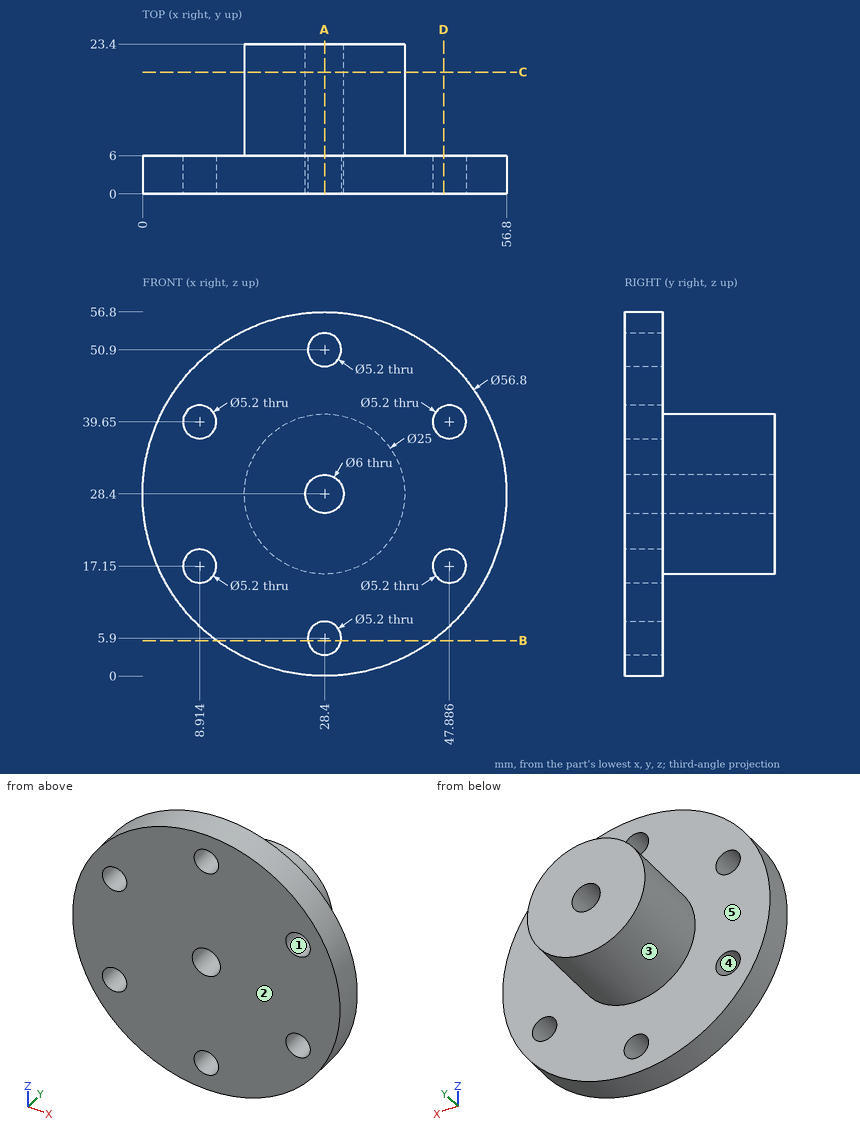
Part print with two shaded views. Sizes in mm from the minimum x, y, z corner. A direction names the side the tool comes from. Round coordinates to 2 decimals unless told otherwise and drop trailing zeros. Loops run counter-clockwise (first coordinate to the right, second up) from the corner with the lowest first, then second, coordinate; pieces in that order, holes last. Notation, with made-up numbers: M 57,23 L 69,23 A14 cw 69,44 Z; hole C -27.5,19 d5. An arc over 180 degrees is marked long. Put each result on its own line as item: value. Start each with the question number.
Item 1: Drop flat-ended pins along their axis: P1, Ø4, axis at y = 3.5, z = 23.5, coming from the -X side; P2, Ø1.5, axis at y = 6.5, z = 38.5, coming from the -X side; P3, Ø6, axis at x = 22, y = 14.5, coming from the -Z side. Give the stop position or say it passes through.
Item 2: Cut at B-B (z = 5.5). List the corners of the cut face in (x, y).
Item 3: Cut at D-D (x = 47). List the corners of the cut face in (y, z) (1 decimal), then the cut area to 3 significant figures.
Item 4: Cut at C-C (y = 19). List the corners of the cut face in (x, z).
Item 5: Mould opens along X. For the marked faces 1, 2 and 3 say: released by +X, released by -X, zero draft, split by the parting line, or undercut.
Item 6: Cut at A-A (x = 28.4). List the corners of the cut face in (y, z), then the cut area to 3 significant figures.
Item 7: Drill centre lines: line 1 along X through (y, z) = (1.4, 17.15) (1 decimal); line 2 along Z through (x, y) = (8.5, 4.5) (1 decimal); line 3 along X through (y, z) = (11.75, 28.5). Where is each one in solid material? Low to high.
Item 8: 3-axis set-ups, long thin cutter, end or side, ignore diameter. For the marked faces 4 and 5: which of +Z, -Z, +X, -X, +Y, -Y reach the whole face in a straight line?
Answer block:
1. P1: x = 0.15
1. P2: x = 1.65
1. P3: z = 16.37
2. outline: M 11.6,0 L 25.83,0 L 25.83,6 L 11.6,6 Z; M 30.97,0 L 45.2,0 L 45.2,6 L 30.97,6 Z
3. outline: M 0,6.9 L 6,6.9 L 6,14.7 L 0,14.7 Z; M 0,19.6 L 6,19.6 L 6,37.2 L 0,37.2 Z; M 0,42.1 L 6,42.1 L 6,49.9 L 0,49.9 Z
3. area: 199 mm2
4. outline: C 28.4,28.4 d25; hole C 28.4,28.4 d6
5. face 1: undercut
5. face 2: zero draft
5. face 3: split by the parting line
6. outline: M 0,0 L 6,0 L 6,3.3 L 0,3.3 Z; M 0,8.5 L 6,8.5 L 6,15.9 L 23.4,15.9 L 23.4,25.4 L 0,25.4 Z; M 0,31.4 L 23.4,31.4 L 23.4,40.9 L 6,40.9 L 6,48.3 L 0,48.3 Z; M 0,53.5 L 6,53.5 L 6,56.8 L 0,56.8 Z
6. area: 573 mm2
7. line 1: 2.3 to 6.3, 11.5 to 45.3, 50.5 to 54.5
7. line 2: 8.1 to 14.6, 19.7 to 37.1, 42.2 to 48.7
7. line 3: 15.9 to 25.4, 31.4 to 40.9
8. face 4: +Y, -Y
8. face 5: +Y
